```python
from build123d import *

# Parameters (mm, degrees)
SKETCH1_W                        = 100
SKETCH1_H                        = 100
BOSS_EXTRUDE1_DEPTH              = 30
SKETCH3_R                        = 10
CUT_EXTRUDE1_DEPTH               = 19
CUT_EXTRUDE1_DEPTH_BACK          = 31
FILLET1_R                        = 10
CHAMFER1_SIZE                    = 5
F_12_0MM_DOWEL_HOLE1_D           = 12
F_12_0MM_DOWEL_HOLE1_CSINK_D     = 12.05
F_12_0MM_DOWEL_HOLE1_CSINK_ANGLE = 90


with BuildPart() as part:
    # Sketch1 → Boss-Extrude1 (new body)
    with BuildSketch(Plane.XY):
        Rectangle(SKETCH1_W, SKETCH1_H)
    extrude(amount=BOSS_EXTRUDE1_DEPTH)

    # Sketch3 → Cut-Extrude1 (cut, two sides)
    with BuildSketch(Plane.XY.offset(30)) as cut_extrude1_sk:
        Circle(SKETCH3_R)
    extrude(amount=CUT_EXTRUDE1_DEPTH, mode=Mode.SUBTRACT)
    extrude(cut_extrude1_sk.sketch, amount=-CUT_EXTRUDE1_DEPTH_BACK, mode=Mode.SUBTRACT)

    # Fillet1
    fillet1_edges = [part.edges().sort_by_distance(p)[0] for p in [
        (-50, 50, 15),
        (50, 50, 15),
        (50, -50, 15),
        (-50, -50, 15),
    ]]
    fillet(fillet1_edges, radius=FILLET1_R)

    # Chamfer1
    chamfer1_edges = [part.edges().sort_by_distance(p)[0] for p in [
        (0, -50, 0),
        (0, -50, 30),
        (-50, 0, 0),
        (0, 50, 0),
        (50, 0, 0),
        (47.071067812, -47.071067812, 0),
        (47.071067812, 47.071067812, 0),
        (-47.071067812, 47.071067812, 0),
        (-47.071067812, -47.071067812, 0),
        (-50, 0, 30),
        (50, 0, 30),
        (0, 50, 30),
        (47.071067812, -47.071067812, 30),
        (47.071067812, 47.071067812, 30),
        (-47.071067812, 47.071067812, 30),
        (-47.071067812, -47.071067812, 30),
    ]]
    chamfer(chamfer1_edges, length=CHAMFER1_SIZE)

    # Ø12.0mm Dowel Hole1 (through all)
    with Locations(Plane(origin=(0, 0, 0), x_dir=(-1, 0, 0), z_dir=(0, 0, -1))):
        with Locations((-36.283625915, 37.887322089), (34.279005699, 37.887322089), (34.279005699, -34.145364351), (-36.283625915, -36.818191306)):
            CounterSinkHole(F_12_0MM_DOWEL_HOLE1_D / 2, F_12_0MM_DOWEL_HOLE1_CSINK_D / 2, counter_sink_angle=F_12_0MM_DOWEL_HOLE1_CSINK_ANGLE)


solid = part.part
```
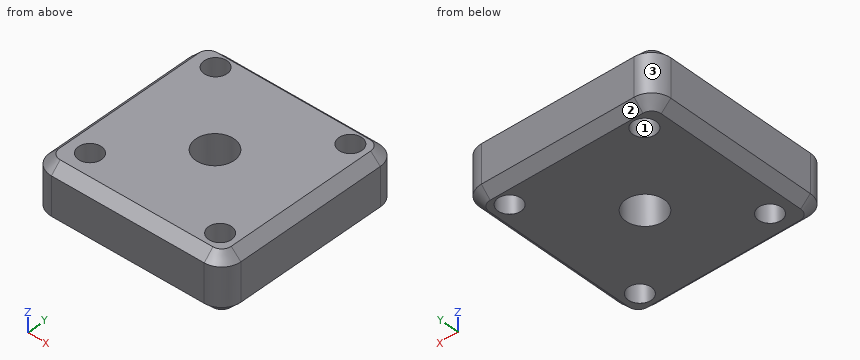
Verification items for the finished model (mm, model axes). Face numbers are marked on the shaded views. Give positions to 0.01 mm unless a question says otherwise; leave off trailing zeros. Write each loop counter-clockwise with the first axis right and the second up, starting at its lowest first coordinate (ties: lowest second). Pieces come first, ordered by that corner, then holes. Notation, with made-up numbers: M 64,8 L 77,8 A11 ccw 77,13 Z; hole C 4,-38.5 d6. An arc over 180 degrees is marked long. One line per question, with ' | ' between items.
1) Thickness scan on line 1 along Y through (x, z) = (0, 22.75); line 2 along Y through (x, z) = (-31.5, 23); line 3 along X through (y, z) = (-40.5, 23). Record the ranges inside material, lowest first. Write a range as [from, to].
Result:
line 1: y = [-50, -10], [10, 50] | line 2: y = [-50, -39.46], [-28.83, 32.57], [43.2, 50] | line 3: x = [-49.99, 31.55], [41.02, 49.99]
2) Section check A-A on x = 0. Enter the section's corners in (y, z).
Result:
outline: M -50,5 L -45,0 L -10,0 L -10,30 L -45,30 L -50,25 Z; M 10,0 L 45,0 L 50,5 L 50,25 L 45,30 L 10,30 Z
3) Mould release check, pull along X, two halves, no side actions. Record for the marked faces 1, 2 and 3: released by +X, released by -X, zero draft, split by the parting line, or undercut.
Result:
face 1: undercut | face 2: zero draft | face 3: released by -X
4) Section check C-C on x = -14. Enter the section's corners in (y, z).
Result:
outline: M -50,5 L -45,0 L 45,0 L 50,5 L 50,25 L 45,30 L -45,30 L -50,25 Z
5) Section check D-D on z = 11.25. Enter the section's corners in (x, y), plus the area to 3 significant figures.
Result:
outline: M -50,-40 A10 ccw -40,-50 L 40,-50 A10 ccw 50,-40 L 50,40 A10 ccw 40,50 L -40,50 A10 ccw -50,40 Z; hole C -34.28,-34.15 d12; hole C -34.28,37.89 d12; hole C 0,0 d20; hole C 36.28,-36.82 d12; hole C 36.28,37.89 d12 | area: 9,150 mm2
